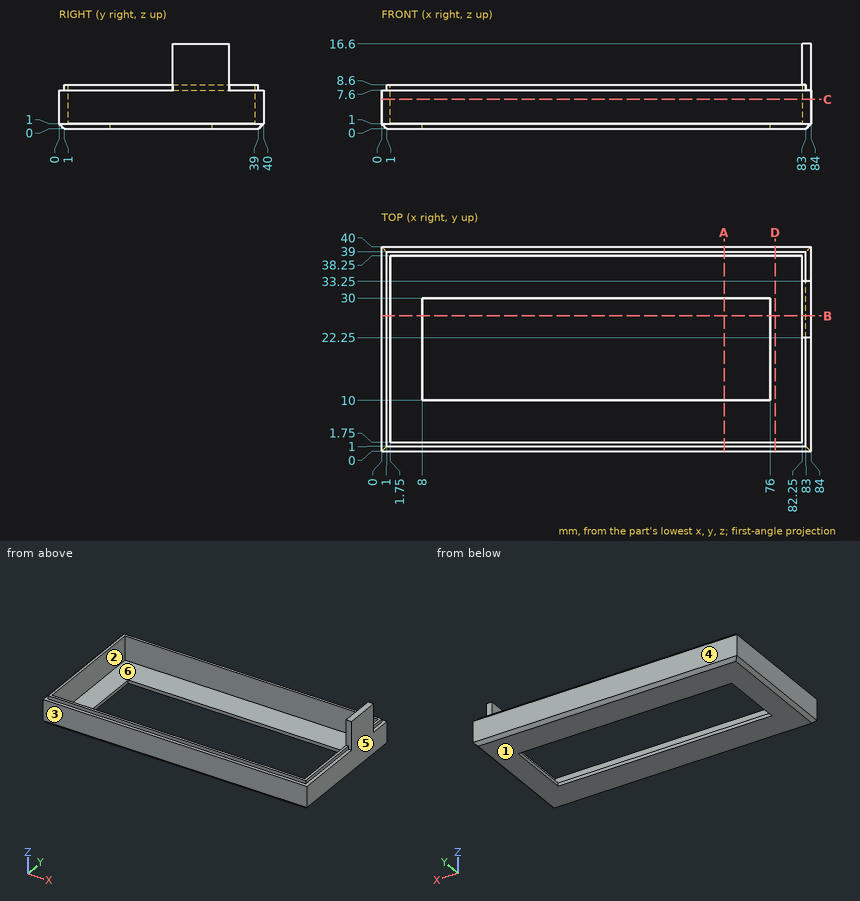
Part print with two shaded views. Sizes in mm from the minimum x, y, z corner. A direction names the side the tool comes from. Give positions to 0.01 mm unless a question says otherwise; leave off trailing zeros. Order: outer loops, then holes, each group sorted by start corner. A loop starts at its lowest first (then second) coordinate and runs counter-clockwise, first axis right, second up. Notation, with made-up numbers: M 23.5,-10.5 L 53.5,-10.5 A22 ccw 53.5,23.5 Z; hole C 70,-7.5 d10. An arc over 180 degrees is marked long. Use one line per item in the form item = value.
1) Saw through at A-A (x = 67). Give the cut face in (y, z), plus the area to 3 significant figures.
Calculated:
outline = M 0,1 L 1,0 L 10,0 L 10,1 L 1.75,1 L 1.75,8.6 L 1,8.6 L 1,7.6 L 0,7.6 Z; M 30,0 L 39,0 L 40,1 L 40,7.6 L 39,7.6 L 39,8.6 L 38.25,8.6 L 38.25,1 L 30,1 Z
area = 43.6 mm2
2) Saw through at B-B (y = 26.5). Give the cut face in (x, z), plus the area to 3 significant figures.
Calculated:
outline = M 0,1 L 1,0 L 8,0 L 8,1 L 1.75,1 L 1.75,8.6 L 1,8.6 L 1,7.6 L 0,7.6 Z; M 76,0 L 83,0 L 84,1 L 84,16.6 L 82.25,16.6 L 82.25,1 L 76,1 Z
area = 54.6 mm2
3) Probe probe 1 along X at (y, z) = (9.5, 7); probe 2 along Y at (x, z) = (7, 1.25); probe 3 along Y at (x, z) = (30.5, 8.5). List the from-to ranges inside material, lowest first.
Calculated:
probe_1 = 0 to 1.75, 82.25 to 84
probe_2 = 0 to 1.75, 38.25 to 40
probe_3 = 1 to 1.75, 38.25 to 39
4) Tool access for the marked faces 5 and 6: list every direction of +Z, -Z, +X, -X, +Y, -Y with a clear straight run to the whole face (end or side of a thin tool).
Calculated:
face_5 = +Z, -Z, +X, +Y, -Y
face_6 = +Z
5) Drop flat-ended pins along their axis: pin 1 (0.5 mm diameter, centred on y = 22, z = 0.5, fed in from -X); pin 2 (0.8 mm diameter, centred on x = 22.5, z = 8.5, fed in from +Y); pin 3 (6 mm diameter, centred on x = 55.5, z = 12, fed in from -Y); pin 4 (10 mm diameter, centred on x = 60.5, y = 27.5, fed in from +Z). Give the stop position or say it passes through.
Calculated:
pin_1 = 0.25
pin_2 = 39
pin_3 = through
pin_4 = 1
6) Saw through at D-D (x = 77). Give the cut face in (y, z).
Calculated:
outline = M 0,1 L 1,0 L 39,0 L 40,1 L 40,7.6 L 39,7.6 L 39,8.6 L 38.25,8.6 L 38.25,1 L 1.75,1 L 1.75,8.6 L 1,8.6 L 1,7.6 L 0,7.6 Z
7) Saw through at C-C (z = 5.75). Give the cut face in (x, y), plus the area to 3 significant figures.
Calculated:
outline = M 0,0 L 84,0 L 84,40 L 0,40 Z; hole M 1.75,1.75 L 82.25,1.75 L 82.25,38.25 L 1.75,38.25 Z
area = 422 mm2
8) Two-plate mould, pull along Y, no slides. Class the marked faces 1, 2, 3 and 4: released by +Y, released by -Y, zero draft, split by the parting line, or undercut.
Calculated:
face_1 = zero draft
face_2 = undercut
face_3 = released by -Y
face_4 = released by +Y
